Geometry check sheet. Reference: the model listing, model coordinates, mm. Give positions to 0.01 mm unless a question says otherwise; leave off trailing zeros. Loops run counter-clockwise (first coordinate to the right, second up) from the corner with the lowest first, then second, coordinate; pieces in that order, holes last.
1. Material ranges on L1, parallel to X at y = 13, z = 27; L2, parallel to X at y = 3.25, z = 27; L3, parallel to Z at x = 0, y = 4.5, recorded low to high.
2. Cross-section at B-B, the plane x = 0. Record the cut outline in (y, z).
3. Cross-section at A-A, the plane z = 27. Record the cut outline in (x, y), plus the area to 3 significant figures.
4. Cross-section at C-C, the plane y = 6. Record the cut outline in (x, z).
from build123d import *

# Parameters (mm, degrees)
SKETCH_1_W               = 344
SKETCH_1_H               = 340
EXTRUDE_1_DEPTH          = 18
SKETCH_2_R               = 114.5
CUT_EXTRUDE_1_DEPTH      = 1
CUT_EXTRUDE_1_DEPTH_BACK = 19
SKETCH_3_R               = 128
CUT_EXTRUDE_2_DEPTH      = 8


with BuildPart() as part:
    # Эскиз1 → Бобышка-Вытянуть1 (new body)
    with BuildSketch(Plane(origin=(0, 0, 0), x_dir=(1, 0, 0), z_dir=(0, 1, 0))):
        Rectangle(SKETCH_1_W, SKETCH_1_H)
    extrude(amount=EXTRUDE_1_DEPTH)

    # Эскиз2 → Вырез-Вытянуть1 (cut, two sides)
    with BuildSketch(Plane(origin=(0, 18, 0), x_dir=(1, 0, 0), z_dir=(0, 1, 0))) as cut_extrude_1_sk:
        with Locations((0, -27)):
            Circle(SKETCH_2_R)
    extrude(amount=CUT_EXTRUDE_1_DEPTH, mode=Mode.SUBTRACT)
    extrude(cut_extrude_1_sk.sketch, amount=-CUT_EXTRUDE_1_DEPTH_BACK, mode=Mode.SUBTRACT)

    # Эскиз3 → Вырез-Вытянуть2 (cut)
    with BuildSketch(Plane(origin=(0, 18, 0), x_dir=(1, 0, 0), z_dir=(0, 1, 0))):
        with Locations((0, -27)):
            Circle(SKETCH_3_R)
    extrude(amount=-CUT_EXTRUDE_2_DEPTH, mode=Mode.SUBTRACT)


solid = part.part
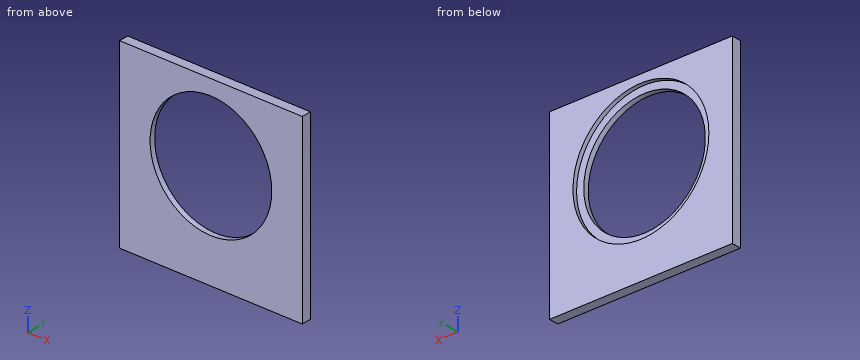
Result:
1. L1: x = -172 to -128, 128 to 172
1. L2: x = -172 to -114.5, 114.5 to 172
1. L3: z = -170 to -87.5, 141.5 to 170
2. outline: (0, -170) - (18, -170) - (18, -101) - (10, -101) - (10, -87.5) - (0, -87.5) - close; (0, 141.5) - (10, 141.5) - (10, 155) - (18, 155) - (18, 170) - (0, 170) - close
3. outline: (-172, 0) - (-114.5, 0) - (-114.5, 10) - (-128, 10) - (-128, 18) - (-172, 18) - close; (114.5, 0) - (172, 0) - (172, 18) - (128, 18) - (128, 10) - (114.5, 10) - close
3. area: 1,850 mm2
4. outline: (-172, -170) - (172, -170) - (172, 170) - (-172, 170) - close; hole circle Ø229 at (0, 27)
